```python
from build123d import *

# Parameters (mm, degrees)
F1_DEPTH = 30
F3_W     = 19.6464200949
F3_H     = 2
F4_DEPTH = 30.001
F2_R     = 5
F5_DEPTH = 30.001
F6_R     = 4
F7_DEPTH = 18.001
F8_DEPTH = 30.001


# Not quite as in the source:
# - a feature names something its author has since deleted; it is built from what else it names


with BuildPart() as f1:
    # F0 (on Right) → F1 (new body)
    with BuildSketch(Plane.YZ):
        Polygon((13.9517640748, 20.9442070276), (24.0209596489, 8.9442070276), (64.0209596489, 8.9442070276), (64.0209596489, 26.9442070276), (0, 26.9442070276), (0, 12.4442070276), (5, 12.4442070276), (10.9517640748, 20.9442070276), align=None)
    extrude(amount=F1_DEPTH)

    # F3 (on face) → F4 (cut, through all)
    with BuildSketch(Plane.YZ.offset(30)):
        with Locations((56.7216197717, 17.9442070276)):
            Rectangle(F3_W, F3_H)
    extrude(amount=-F4_DEPTH, mode=Mode.SUBTRACT)

    # F2 (on face) → F5 (cut, through all)
    with BuildSketch(Plane.YZ.offset(30)):
        with Locations((44.0209596489, 17.9442070276)):
            Circle(F2_R)
    extrude(amount=-F5_DEPTH, mode=Mode.SUBTRACT)

    # F6 (on face) → F7 (cut, through all)
    with BuildSketch(Plane.XY.offset(26.9442070276)):
        with Locations((15, 31.5209596489)):
            Circle(F6_R)
        with Locations((15, 56.5209596489)):
            Circle(F6_R)
    extrude(amount=-F7_DEPTH, mode=Mode.SUBTRACT)

    # F2 (on face) → F8 (cut, through all)
    with BuildSketch(Plane.YZ.offset(30)):
        with Locations((44.0209596489, 17.9442070276)):
            Circle(F2_R)
    extrude(amount=-F8_DEPTH, mode=Mode.SUBTRACT)


solid = f1.part
```
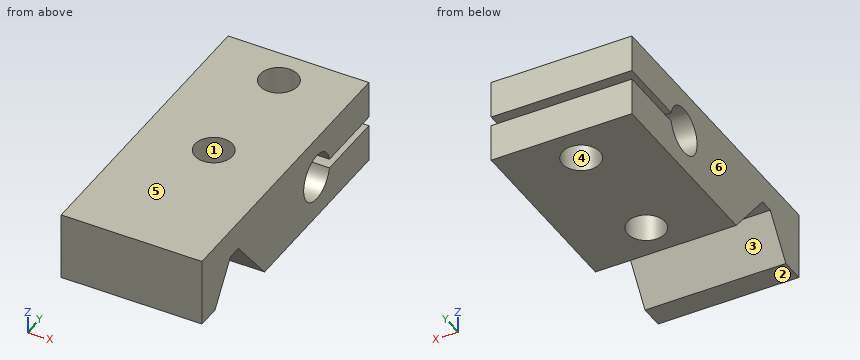
The listing builds one solid part. Answer for the finished solid, in the listing's coordinates (mm). Face numbers are marked on the shaded views. A direction names the side the tool comes from. Give positions to 0.01 mm unless a question says otherwise; leave off trailing zeros. Order: outer loops, then holes, each group sorted by start corner. A loop starts at its lowest first (then second) coordinate and runs counter-clockwise, first axis right, second up. Notation, with made-up numbers: (30.25, 88) - (85.25, 88) arc R8 cw to (85.25, 101) - close; hole circle Ø5 at (65, -16.5). An arc over 180 degrees is marked (long way). Use one line per item in the form item = value. Start each with the question number.
(1) The mould has two halves that part along X. Classify the marked faces 4, 5 and 6: released by +X, released by -X, zero draft, split by the parting line, or undercut.
(2) A cutting plane is placed at A-A, the plane x = 15. Write down the section's boundary in (y, z).
(3) A cutting plane is placed at C-C, the plane y = 45.5. Write down the section's boundary in (x, z), then the cut area to 3 significant figures.
(4) Consider line 1 (Y direction, x = 15, z = 24.25); line 2 (Z direction, x = 8.5, y = 54.5); line 3 (Y direction, x = 15, z = 22). Determine where each line is inside the solid, lowest interval first. Write a range as from..to.
(5) For the marked faces 1, 2 and 3, determine the directions among +Z, -Z, +X, -X, +Y, -Y from which every point of the face is accessible in a straight line to the end or side of a thin tool.
(6) A cutting plane is placed at D-D, the plane x = 2.25. Write down the section's boundary in (y, z).
(7) A cutting plane is placed at B-B, the plane z = 18.25. Write down the section's boundary in (x, y).
(8) Flat-ended cylindrical pins translate along their axes: pin 1 Ø1.5 at (x, y) = (17, 12.5) entering from -Z; pin 2 Ø5.5 at (x, y) = (19.5, 2.5) entering from -Z; pin 3 Ø6.5 at (x, y) = (15, 56.52) entering from -Z. Find the tip coordinate at first contact, or state that the pin passes through.
Ans:
q1.face_4 = undercut
q1.face_5 = zero draft
q1.face_6 = released by -X
q2.outline = (0, 12.44) - (5, 12.44) - (10.95, 20.94) - (13.95, 20.94) - (24.02, 8.94) - (27.52, 8.94) - (27.52, 26.94) - (0, 26.94) - close; (35.52, 8.94) - (52.52, 8.94) - (52.52, 16.94) - (48.92, 16.94) arc R5 cw (long way) to (48.92, 18.94) - (52.52, 18.94) - (52.52, 26.94) - (35.52, 26.94) - close; (60.52, 8.94) - (64.02, 8.94) - (64.02, 16.94) - (60.52, 16.94) - close; (60.52, 18.94) - (64.02, 18.94) - (64.02, 26.94) - (60.52, 26.94) - close
q3.outline = (0, 8.94) - (30, 8.94) - (30, 13.17) - (0, 13.17) - close; (0, 22.72) - (30, 22.72) - (30, 26.94) - (0, 26.94) - close
q3.area = 253 mm^2
q4.line_1 = 0..27.52, 35.52..52.52, 60.52..64.02
q4.line_2 = 8.94..16.94, 18.94..26.94
q4.line_3 = 0..27.52, 35.52..41.1, 46.95..52.52, 60.52..64.02
q5.face_1 = +Z, -Z
q5.face_2 = -Z, +X, -X, -Y
q5.face_3 = -Z, +X, -X
q6.outline = (0, 12.44) - (5, 12.44) - (10.95, 20.94) - (13.95, 20.94) - (24.02, 8.94) - (64.02, 8.94) - (64.02, 16.94) - (48.92, 16.94) arc R5 cw (long way) to (48.92, 18.94) - (64.02, 18.94) - (64.02, 26.94) - (0, 26.94) - close
q7.outline = (0, 0) - (30, 0) - (30, 9.07) - (0, 9.07) - close; (0, 16.21) - (30, 16.21) - (30, 39.03) - (0, 39.03) - close; hole circle Ø8 at (15, 31.52)
q8.pin_1 = 20.94
q8.pin_2 = 12.44
q8.pin_3 = through
